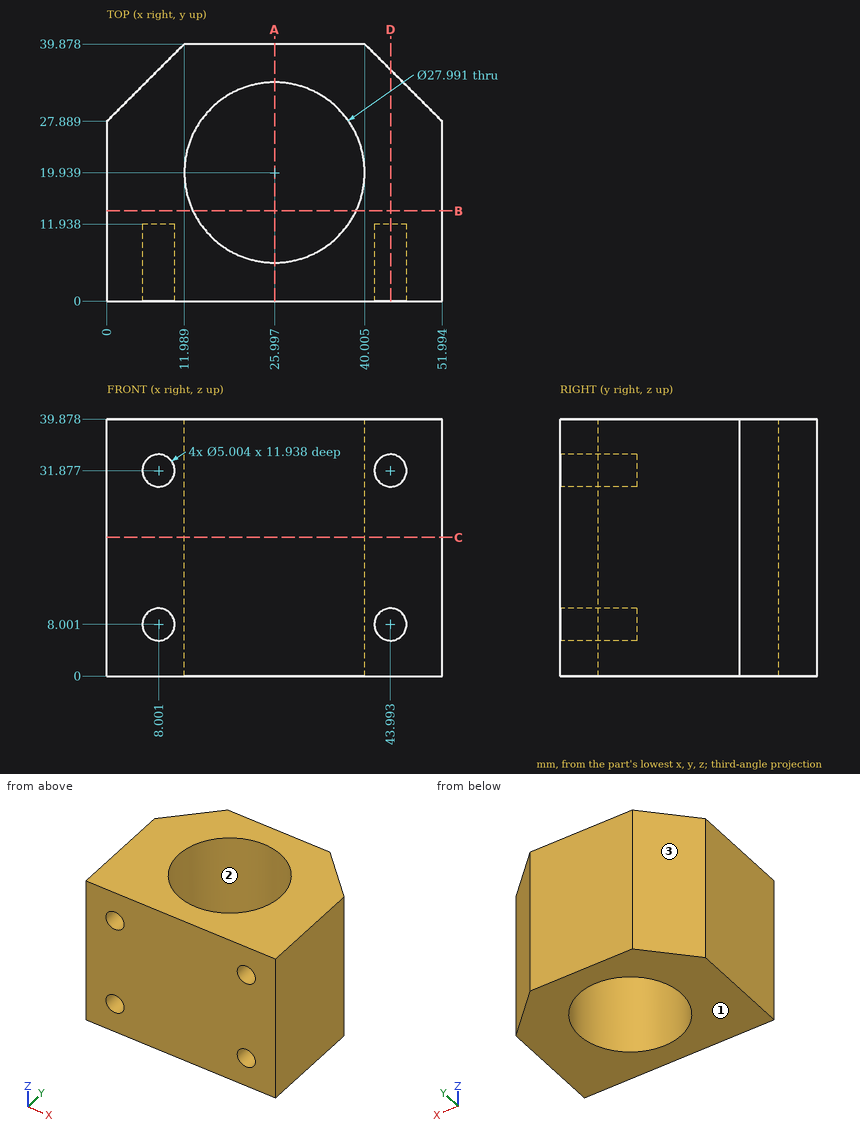
Design review of the part shown in the three views and the two pictorial views. Dimensions are in mm from the part's minimum x, y and z. Round coordinates to 2 decimals unless told otherwise and drop trailing zeros. Loops run counter-clockwise (first coordinate to the right, second up) from the corner with the lowest first, then second, coordinate; pieces in that order, holes last. Notation, with made-up numbers: M -26,57 L -22,57 A31 cw -22,96 Z; hole C -36.5,89 d9. An arc over 180 degrees is marked long. Put each result on its own line as item: value.
Q1. For pin 1 (3 mm diameter, centred on x = 36, y = 25.5, fed in from -Z); pin 2 (4.5 mm diameter, centred on x = 8.001, z = 31.877, fed in from +Y); pin 3 (4 mm diameter, centred on x = 43.99, z = 31.88, fed in from +Y); pin 4 (1.5 mm diameter, centred on y = 29.5, z = 20.5, fed in from -X), all flat-tipped, find the tip position at first contact; note any pin that passes through.
Result set:
pin 1: passes through
pin 2: stops at y = 38.14
pin 3: stops at y = 37.89
pin 4: stops at x = 0.86
Q2. Consider section C-C, the plane z = 21.5. Give the boundary of the cut face in (x, y) (1 decimal).
Result set:
outline: M 0,0 L 52,0 L 52,27.9 L 40,39.9 L 12,39.9 L 0,27.9 Z; hole C 26,19.9 d28
Q3. Mouldability with a two-part tool opening along Y and no side actions: class the marked faces 1, 2 and 3 as released by +Y, released by -Y, zero draft, split by the parting line, or undercut.
Result set:
face 1: zero draft
face 2: undercut
face 3: released by +Y
Q4. Consider section B-B, the plane y = 14. Give the boundary of the cut face in (x, z), then the cut area to 3 significant figures.
Result set:
outline: M 0,0 L 13.32,0 L 13.32,39.88 L 0,39.88 Z; M 38.67,0 L 51.99,0 L 51.99,39.88 L 38.67,39.88 Z
area: 1,060 mm²
Q5. To check wall thickness, follow L1, parallel to X at y = 20.5, z = 21; L2, parallel to X at y = 3.5, z = 8.5 (1 decimal); L3, parallel to X at y = 8, z = 31.5 (1 decimal). State the ranges of each line that lie inside material, in increasing order.
Result set:
L1: x = 0 to 12.01, 39.98 to 51.99
L2: x = 0 to 5.5, 10.5 to 41.5, 46.4 to 52
L3: x = 0 to 5.5, 10.5 to 18.7, 33.3 to 41.5, 46.5 to 52
Q6. Consider section D-D, the plane x = 44. Give the boundary of the cut face in (y, z) (1 decimal), then the cut area to 3 significant figures.
Result set:
outline: M 0,0 L 35.9,0 L 35.9,39.9 L 0,39.9 L 0,34.4 L 11.9,34.4 L 11.9,29.4 L 0,29.4 L 0,10.5 L 11.9,10.5 L 11.9,5.5 L 0,5.5 Z
area: 1,310 mm²
Q7. Consider section A-A, the plane x = 26. Give the boundary of the cut face in (y, z).
Result set:
outline: M 0,0 L 5.94,0 L 5.94,39.88 L 0,39.88 Z; M 33.93,0 L 39.88,0 L 39.88,39.88 L 33.93,39.88 Z
